Part model, mm, in its own coordinate system. Face numbers are marked on the shaded views. A direction names the side the tool comes from. Give positions to 0.01 mm unless a question says otherwise; leave off trailing zeros. Order: outer loops, then holes, each group sorted by start corner. A loop starts at its lowest first (then second) coordinate and runs counter-clockwise, first axis right, second up.
1. Mould opens along Y. For the marked faces 1, 2 and 3 say: +Y half, -Y half, draft (parallel to the pull), parting line (faces both ways), or undercut.
2. Slice it at B-B on x = 6. List the corners of the cut face in (y, z), and give its area (3 significant figures).
3. Which spindle directions (+Z, -Z, +X, -X, +Y, -Y) get a long thin tool onto all of the face, cutting with end or side? Do the marked faces 4 and 5. Say none if no direction does.
4. Slice it at C-C on z = 6.5. Give the number of separate pieces and of enclosed holes in the cut face, and give its area (3 significant figures).
5. Probe line 1 (Y direction, x = -16.5, z = 4.5); line 2 (X direction, y = 4, z = 5.75); line 3 (Y direction, x = 17, z = 4.75). List the from-to ranges inside material, lowest first.
6. Drop flat-ended pins along their axis: pin 1 Ø12 at (x, y) = (-2, -5) entering from +Z; pin 2 Ø1.2 at (x, y) = (17, -22) entering from +Z; pin 3 Ø0.8 at (x, z) = (-17.5, 5.5) entering from -Y. Give the stop position or say it passes through.
7. Slice it at A-A on y = -11. List the corners of the cut face in (x, z), and give its area (3 significant figures).
from build123d import *

# Parameters (mm, degrees)
BOSS_EXTRUDE1_DEPTH = 9.6
CUT_EXTRUDE1_START  = 9.6
CUT_EXTRUDE1_DEPTH  = 1.6
CUT_EXTRUDE2_START  = 9.6
CUT_EXTRUDE2_DEPTH  = 8.1
CUT_EXTRUDE3_START  = 9.6
SKETCH5_R           = 1.25
CUT_EXTRUDE3_DEPTH  = 8.1
FILLET2_R           = 1
FILLET3_R           = 3


with BuildPart() as part:
    # Sketch2 → Boss-Extrude1 (new body)
    with BuildSketch(Plane.XY):
        with BuildLine():
            Line((21, 21.5), (21, -21.5))
            ThreePointArc((21, -21.5), (19.681980515, -24.681980515), (16.5, -26))
            Line((16.5, -26), (-16.5, -26))
            ThreePointArc((-16.5, -26), (-19.681980515, -24.681980515), (-21, -21.5))
            Line((-21, -21.5), (-21, 21.5))
            ThreePointArc((-21, 21.5), (-19.681980515, 24.681980515), (-16.5, 26))
            Line((-16.5, 26), (16.5, 26))
            ThreePointArc((16.5, 26), (19.681980515, 24.681980515), (21, 21.5))
        make_face()
    extrude(amount=BOSS_EXTRUDE1_DEPTH)

    # Sketch3 → Cut-Extrude1 (cut)
    with BuildSketch(Plane.XY.offset(CUT_EXTRUDE1_START)):
        with BuildLine():
            Line((-20, 21.5), (-20, -21.5))
            ThreePointArc((-20, -21.5), (-18.974873734, -23.974873734), (-16.5, -25))
            Line((-16.5, -25), (16.5, -25))
            ThreePointArc((16.5, -25), (18.974873734, -23.974873734), (20, -21.5))
            Line((20, -21.5), (20, 21.5))
            ThreePointArc((20, 21.5), (18.974873734, 23.974873734), (16.5, 25))
            Line((16.5, 25), (-16.5, 25))
            ThreePointArc((-16.5, 25), (-18.974873734, 23.974873734), (-20, 21.5))
        make_face()
    extrude(amount=-CUT_EXTRUDE1_DEPTH, mode=Mode.SUBTRACT)

    # Sketch4 → Cut-Extrude2 (cut)
    with BuildSketch(Plane.XY.offset(CUT_EXTRUDE2_START)):
        with BuildLine():
            Line((-12.5, -21.5), (-12.5, -24))
            Line((-12.5, -24), (12.5, -24))
            Line((12.5, -24), (12.5, -21.5))
            ThreePointArc((12.5, -21.5), (13.671572875, -18.671572875), (16.5, -17.5))
            Line((16.5, -17.5), (19, -17.5))
            Line((19, -17.5), (19, 17.5))
            Line((19, 17.5), (16.5, 17.5))
            ThreePointArc((16.5, 17.5), (13.671572875, 18.671572875), (12.5, 21.5))
            Line((12.5, 21.5), (12.5, 24))
            Line((12.5, 24), (-12.5, 24))
            Line((-12.5, 24), (-12.5, 21.5))
            ThreePointArc((-12.5, 21.5), (-13.671572875, 18.671572875), (-16.5, 17.5))
            Line((-16.5, 17.5), (-19, 17.5))
            Line((-19, 17.5), (-19, -17.5))
            Line((-19, -17.5), (-16.5, -17.5))
            ThreePointArc((-16.5, -17.5), (-13.671572875, -18.671572875), (-12.5, -21.5))
        make_face()
    extrude(amount=-CUT_EXTRUDE2_DEPTH, mode=Mode.SUBTRACT)

    # Sketch5 → Cut-Extrude3 (cut)
    with BuildSketch(Plane.XY.offset(CUT_EXTRUDE3_START)):
        with Locations((-16.5, 21.5)):
            Circle(SKETCH5_R)
        with Locations((16.5, 21.5)):
            Circle(SKETCH5_R)
        with Locations((-16.5, -21.5)):
            Circle(SKETCH5_R)
        with Locations((16.5, -21.5)):
            Circle(SKETCH5_R)
    extrude(amount=-CUT_EXTRUDE3_DEPTH, mode=Mode.SUBTRACT)

    # Fillet2
    fillet2_edges = [part.edges().sort_by_distance(p)[0] for p in [
        (13.671572875, -18.671572875, 1.5),
        (12.5, -22.75, 1.5),
        (0, -24, 1.5),
        (12.5, -24, 4.75),
        (-12.5, -22.75, 1.5),
        (-12.5, -24, 4.75),
        (-13.671572875, -18.671572875, 1.5),
        (-17.75, -17.5, 1.5),
        (-19, 0, 1.5),
        (-19, -17.5, 4.75),
        (-17.75, 17.5, 1.5),
        (-19, 17.5, 4.75),
        (-13.671572875, 18.671572875, 1.5),
        (-12.5, 22.75, 1.5),
        (0, 24, 1.5),
        (-12.5, 24, 4.75),
        (12.5, 22.75, 1.5),
        (12.5, 24, 4.75),
        (13.671572875, 18.671572875, 1.5),
        (17.75, 17.5, 1.5),
        (19, 0, 1.5),
        (19, 17.5, 4.75),
        (17.75, -17.5, 1.5),
        (19, -17.5, 4.75),
    ]]
    fillet(fillet2_edges, radius=FILLET2_R)

    # Fillet3
    fillet3_edges = [part.edges().sort_by_distance(p)[0] for p in [
        (-21, 0, 0),
        (-19.681980515, 24.681980515, 0),
        (0, 26, 0),
        (19.681980515, 24.681980515, 0),
        (21, 0, 0),
        (19.681980515, -24.681980515, 0),
        (0, -26, 0),
        (-19.681980515, -24.681980515, 0),
    ]]
    fillet(fillet3_edges, radius=FILLET3_R)


solid = part.part
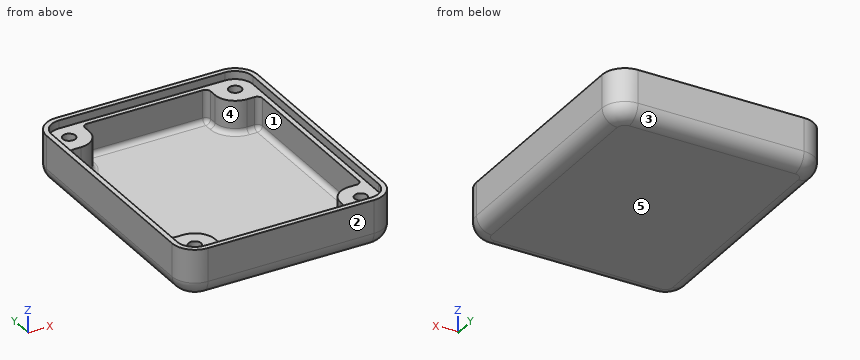
Data:
1. face 1: undercut
1. face 2: -Y half
1. face 3: +Y half
2. outline: (-26, 3) arc R3 ccw to (-23, 0) - (23, 0) arc R3 ccw to (26, 3) - (26, 9.6) - (25, 9.6) - (25, 8) - (24, 8) - (24, 2.5) arc R1 cw to (23, 1.5) - (-23, 1.5) arc R1 cw to (-24, 2.5) - (-24, 8) - (-25, 8) - (-25, 9.6) - (-26, 9.6) - close
2. area: 104 mm2
3. face 4: +Z
3. face 5: -Z, +X, -X, +Y, -Y
4. separate pieces: 1
4. enclosed holes: 5
4. area: 480 mm2
5. line 1: y = -26 to -22.75, -20.25 to -17.5, 17.5 to 20.25, 22.75 to 26
5. line 2: x = -21 to -19, 19 to 21
5. line 3: y = -25.97 to -22.65, -20.35 to -17.5, 17.5 to 20.35, 22.65 to 25.97
6. pin 1: stops at z = 1.5
6. pin 2: stops at z = 8
6. pin 3: stops at y = -25.96
7. outline: (-21, 3) arc R3 ccw to (-18, 0) - (18, 0) arc R3 ccw to (21, 3) - (21, 9.6) - (20, 9.6) - (20, 8) - (19, 8) - (19, 2.5) arc R1 cw to (18, 1.5) - (-18, 1.5) arc R1 cw to (-19, 2.5) - (-19, 8) - (-20, 8) - (-20, 9.6) - (-21, 9.6) - close
7. area: 88.8 mm2
